Check sheet for the modelled part. Datum: model origin and axes. Units: mm. Face numbers are marked on the shaded views. A direction names the side the tool comes from. Round coordinates to 2 decimals unless told otherwise and drop trailing zeros. Write each loop counter-clockwise with the first axis right and the second up, starting at its lowest first coordinate (ties: lowest second). Pieces come first, ordered by that corner, then holes.
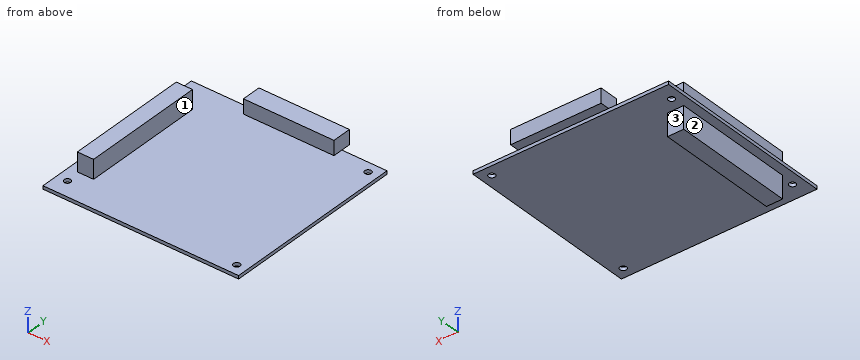
from build123d import *

# Parameters (mm, degrees)
SKETCH1_W                    = 96.0628
SKETCH1_H                    = 90.3478
PCB_DEPTH                    = 1.6256
SKETCH5_R                    = 1.5875
PCB_HOLES_DEPTH              = 66.957101229
PCI_104_CONNECTOR_DEPTH      = 9.2964
PCI_104_CONNECTOR_DEPTH_BACK = 12.6238
SKETCH2_W                    = 7.9756
SKETCH2_H                    = 60.2234
SKETCH6_W                    = 44.45
SKETCH6_H                    = 9.398
PCB_EDGE_CONNS_DEPTH         = 7.112


with BuildPart() as part:
    # Sketch1 → PCB (new body)
    with BuildSketch(Plane.XY):
        Rectangle(SKETCH1_W, SKETCH1_H)
    extrude(amount=PCB_DEPTH)

    # Sketch5 → PCB_Holes (cut, through all)
    with BuildSketch(Plane.XY.offset(1.6256)):
        with Locations((-42.7736, 36.83)):
            Circle(SKETCH5_R)
        with Locations((42.9514, 40.005)):
            Circle(SKETCH5_R)
        with Locations((42.9514, -40.005)):
            Circle(SKETCH5_R)
        with Locations((-42.7736, -36.83)):
            Circle(SKETCH5_R)
    extrude(amount=-PCB_HOLES_DEPTH, mode=Mode.SUBTRACT)

    # Sketch2 → PCI-104_Connector (add, two sides: drawn at the far end of the back side and taken through both)
    with BuildSketch(Plane.XY.offset(1.6256).offset(-PCI_104_CONNECTOR_DEPTH_BACK)):
        with Locations((-39.6494, 0.4064)):
            Rectangle(SKETCH2_W, SKETCH2_H)
    extrude(amount=PCI_104_CONNECTOR_DEPTH + PCI_104_CONNECTOR_DEPTH_BACK)

    # Sketch6 → PCB_Edge_Conns (add)
    with BuildSketch(Plane.XY.offset(1.6256)):
        with Locations((3.6576, 45.0469)):
            Rectangle(SKETCH6_W, SKETCH6_H)
    extrude(amount=PCB_EDGE_CONNS_DEPTH)


solid = part.part
1. Scan lines: line 1 along X through (y, z) = (-14.5, -8.5); line 2 along Y through (x, z) = (15.5, 7.25); line 3 along Z through (x, y) = (-12, 35). Record each from-to range of solid material in increasing order.
2. Sectioned sample at D-D, the plane y = 19. Enter the section's corners in (x, z), plus the area to 3 significant figures.
3. Set-up check for the marked faces 1, 2 and 3: record each of +Z, -Z, +X, -X, +Y, -Y from which the full face is reachable in a straight line by a thin tool's end or side.
4. Go/stop test with flat-tipped pins: pin 1 (4 mm diameter, centred on y = -23, z = -7.5, fed in from -X); pin 2 (2 mm diameter, centred on y = 46, z = 4.5, fed in from -X); pin 3 (10 mm diameter, centred on y = 4.5, z = 8.5, fed in from +X); pin 4 (5 mm diameter, centred on x = 2.5, z = 4, fed in from -Y). Record where each tip stops, or that it passes through.
5. Sectioned sample at B-B, the plane y = 36.83. Enter the section's corners in (x, z).
6. Sectioned sample at C-C, the plane x = 11.5. Enter the section's corners in (y, z), plus the area to 3 significant figures.
7. Sectioned sample at A-A, the plane z = 3. Enter the section's corners in (x, y).
Computed values:
1. line 1: x = -43.64 to -35.66
1. line 2: y = 40.35 to 49.75
1. line 3: z = 0 to 1.63
2. outline: (-48.03, 0) - (-43.64, 0) - (-43.64, -11) - (-35.66, -11) - (-35.66, 0) - (48.03, 0) - (48.03, 1.63) - (-35.66, 1.63) - (-35.66, 10.92) - (-43.64, 10.92) - (-43.64, 1.63) - (-48.03, 1.63) - close
2. area: 318 mm2
3. face 1: +Z, +X, +Y, -Y
3. face 2: -Z, -X, +Y, -Y
3. face 3: -Z, +X, -X, +Y
4. pin 1: stops at x = -43.64
4. pin 2: stops at x = -18.57
4. pin 3: stops at x = -35.66
4. pin 4: stops at y = -45.17
5. outline: (-48.03, 0) - (-44.36, 0) - (-44.36, 1.63) - (-48.03, 1.63) - close; (-41.19, 0) - (48.03, 0) - (48.03, 1.63) - (-41.19, 1.63) - close
6. outline: (-45.17, 0) - (45.17, 0) - (45.17, 1.63) - (49.75, 1.63) - (49.75, 8.74) - (40.35, 8.74) - (40.35, 1.63) - (-45.17, 1.63) - close
6. area: 214 mm2
7. outline: (-43.64, -29.71) - (-35.66, -29.71) - (-35.66, 30.52) - (-43.64, 30.52) - close; (-18.57, 40.35) - (25.88, 40.35) - (25.88, 49.75) - (-18.57, 49.75) - close
